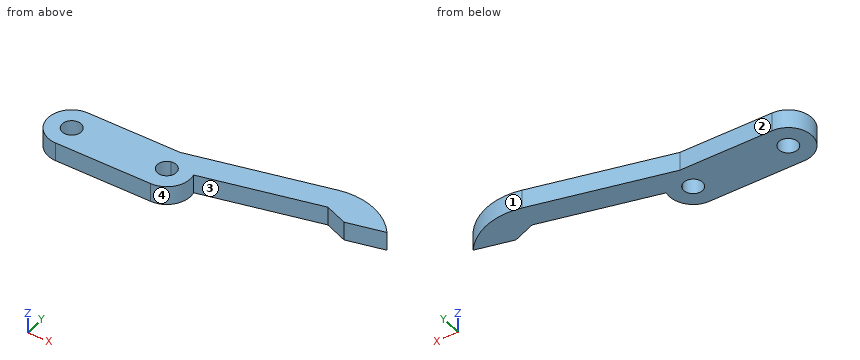
```python
from build123d import *

# Parameters (mm, degrees)
EXTRUDE_1_DEPTH     = 4
SKETCH_2_R          = 2
CUT_EXTRUDE_1_DEPTH = 4
EXTRUDE_3_DEPTH     = 4


with BuildPart() as part:
    # 草图1 → 凸台-拉伸1 (new body)
    with BuildSketch(Plane.XY):
        with BuildLine():
            Line((-10, 5), (10, 5))
            ThreePointArc((10, 5), (15, 0), (10, -5))
            Line((10, -5), (-10, -5))
            ThreePointArc((-10, -5), (-15, 0), (-10, 5))
        make_face()
    extrude(amount=EXTRUDE_1_DEPTH)

    # 草图2 → 切除-拉伸1 (cut)
    with BuildSketch(Plane.XY.offset(4)):
        with Locations((-10, 0)):
            Circle(SKETCH_2_R)
        with Locations((10, 0)):
            Circle(SKETCH_2_R)
    extrude(amount=-CUT_EXTRUDE_1_DEPTH, mode=Mode.SUBTRACT)

    # 草图3 → 凸台-拉伸3 (add)
    with BuildSketch(Plane.XY.offset(4)):
        with BuildLine():
            Line((11.946050783, 0.461396089), (39.19076174, 6.920941341))
            Line((39.19076174, 6.920941341), (43.837655244, 5.075303033))
            Line((43.837655244, 5.075303033), (51.621858375, 6.920887391))
            ThreePointArc((51.621858375, 6.920887391), (45.551115726, 11.368196193), (38.037271516, 11.786068297))
            Line((38.037271516, 11.786068297), (8.846509777, 4.865126957))
            Line((8.846509777, 4.865126957), (9.538603911, 1.946050783))
            ThreePointArc((9.538603911, 1.946050783), (11.049809401, 1.702322009), (11.946050783, 0.461396089))
        make_face()
    extrude(amount=-EXTRUDE_3_DEPTH)


solid = part.part
```
Can you work these out from the model? Positions are in its coordinate system, mm. Face numbers are marked on the shaded views. Give positions to 0.01 mm unless a question says otherwise; leave off trailing zeros. Order: outer loops, then holes, each group sorted by start corner. A loop starts at its lowest first (then second) coordinate and runs counter-clockwise, first axis right, second up. Notation, with made-up numbers: (-39.75, 43.5) - (16.25, 43.5) arc R29 ccw to (16.25, 72.5) - close; hole circle Ø11 at (-27, 79.25). An arc over 180 degrees is marked (long way). Use a Markdown table: item, result. Add a question column.
Q1. If we section it at B-B on x = 13.5: Write out the boundary of the cut face in (y, z).
Q2. If we mould it in two halves opening along X, with no side actions, what happens to the marked faces 1, 2, 3 and 4? For each: released by +X, released by -X, zero draft, split by the parting line, or undercut.
Q3. I'm going to push flat-ended pins straight in: pin 1 (1 mm diameter, centred on x = 21.5, y = 8.5, fed in from +Z); pin 2 (5 mm diameter, centred on x = 10, y = 0, fed in from -Z). Where does each tip first touch, or does it pass through?
Q4. If we section it at A-A on y = 4.25: Write out the boundary of the cut face in (x, z), plus the area to 3 significant figures.
Q5. Please list where these lines run through material, in increasing order: line 1 along Y through (x, z) = (-10, 1); line 2 along Y through (x, z) = (-5.5, 0.2); line 3 along Y through (x, z) = (11, 1.4).
Answers follow:
| question | item | result |
|---|---|---|
| 1 | outline | (-3.57, 0) - (5.97, 0) - (5.97, 4) - (-3.57, 4) - close |
| 2 | face 1 | split by the parting line |
| 2 | face 2 | zero draft |
| 2 | face 3 | undercut |
| 2 | face 4 | released by +X |
| 3 | pin 1 | passes through |
| 3 | pin 2 | stops at z = 0 |
| 4 | outline | (-12.63, 0) - (27.93, 0) - (27.93, 4) - (-12.63, 4) - close |
| 4 | area | 162 mm^2 |
| 5 | line 1 | y = -5 to -2, 2 to 5 |
| 5 | line 2 | y = -5 to 5 |
| 5 | line 3 | y = -4.9 to -1.73, 1.73 to 5.38 |
